Build history of the part. All positions in model axes, mm. Face numbers are marked on the shaded views. Round coordinates to 2 decimals unless told otherwise and drop trailing zeros. Order: outer loops, then holes, each group sorted by start corner. A loop starts at its lowest first (then second) coordinate and runs counter-clockwise, first axis right, second up. Notation, with made-up numbers: (-8.75, -35) -> (6.25, -35) arc R7 ccw to (6.25, -31) -> close; hole circle Ø8 at (33.25, 61). An arc over 180 degrees is marked (long way). Answer as CSV lines item,"result". Start each with the question number.
```python
from build123d import *

# Parameters (mm, degrees)
SKETCH1_R           = 5.159375
BASE_EXTRUDE_DEPTH  = 6.35
SKETCH2_R           = 20.6375
BOSS_EXTRUDE1_DEPTH = 22.225
BOSS_EXTRUDE1_TAPER = 3
SKETCH3_R           = 9.525
CUT_EXTRUDE1_DEPTH  = 52.219943931
SKETCH4_R           = 11.1125
SKETCH4_R_2         = 9.525
BOSS_EXTRUDE2_DEPTH = 0.0254
BOSS_EXTRUDE2_DRAFT = 15
SKETCH5_R           = 11.1125
CUT_EXTRUDE2_DEPTH  = 0.79375
FILLET1_R           = 1.42875


with BuildPart() as part:
    # Sketch1 → Base-Extrude (new body)
    with BuildSketch(Plane(origin=(0, 0, 0), x_dir=(0, 0, -1), z_dir=(1, 0, 0))):
        with BuildLine():
            Line((-7.223125, -19.332171929), (-35.08375, -8.92254089))
            ThreePointArc((-35.08375, -8.92254089), (-41.275, 0), (-35.08375, 8.92254089))
            Line((-35.08375, 8.92254089), (-7.223125, 19.332171929))
            ThreePointArc((-7.223125, 19.332171929), (0, 20.6375), (7.223125, 19.332171929))
            Line((7.223125, 19.332171929), (35.08375, 8.92254089))
            ThreePointArc((35.08375, 8.92254089), (41.275, 0), (35.08375, -8.92254089))
            Line((35.08375, -8.92254089), (7.223125, -19.332171929))
            ThreePointArc((7.223125, -19.332171929), (0, -20.6375), (-7.223125, -19.332171929))
        make_face()
        with Locations((-31.75, 0)):
            Circle(SKETCH1_R, mode=Mode.SUBTRACT)
        with Locations((31.75, 0)):
            Circle(SKETCH1_R, mode=Mode.SUBTRACT)
    extrude(amount=-BASE_EXTRUDE_DEPTH)

    # Sketch2 → Boss-Extrude1 (add)
    with BuildSketch(Plane.ZY):
        Circle(SKETCH2_R)
    extrude(amount=BOSS_EXTRUDE1_DEPTH, taper=BOSS_EXTRUDE1_TAPER)

    # Sketch3 → Cut-Extrude1 (cut, through all)
    with BuildSketch(Plane.ZY.offset(22.225)):
        Circle(SKETCH3_R)
    extrude(amount=-CUT_EXTRUDE1_DEPTH, mode=Mode.SUBTRACT)


with BuildPart() as boss_extrude2_tool:
    # Sketch4 → Boss-Extrude2 (with draft: the straight prism first)
    with BuildSketch(Plane.ZY.offset(22.225)):
        Circle(SKETCH4_R)
        Circle(SKETCH4_R_2, mode=Mode.SUBTRACT)
    extrude(amount=BOSS_EXTRUDE2_DEPTH)
    # Boss-Extrude2: the draft: its side faces are tilted about the plane it starts from
    boss_extrude2_sides = [boss_extrude2_tool.faces().sort_by_distance(p)[0] for p in [
        (-22.2377, 0, -11.1125),
        (-22.2377, 0, -9.525),
    ]]
    draft(boss_extrude2_sides, Plane.ZY.offset(22.225), BOSS_EXTRUDE2_DRAFT)


with BuildPart() as part_1:
    add(part.part)

    # Boss-Extrude2: add boss_extrude2_tool
    add(boss_extrude2_tool.part)

    # Sketch5 → Cut-Extrude2 (cut)
    with BuildSketch(Plane(origin=(0, 0, 0), x_dir=(0, 0, -1), z_dir=(1, 0, 0))):
        Circle(SKETCH5_R)
    extrude(amount=-CUT_EXTRUDE2_DEPTH, mode=Mode.SUBTRACT)

    # Fillet1
    fillet1_edges = [part_1.edges().sort_by_distance(p)[0] for p in [
        (-22.225, 0, -19.472737105),
    ]]
    fillet(fillet1_edges, radius=FILLET1_R)


solid = part_1.part
```
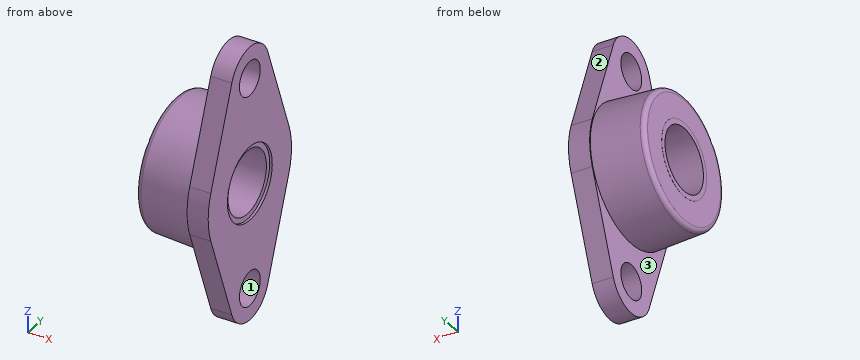
Q1. Two-plate mould, pull along Z, no slides. Class the marked faces 1, 2 and 3: +Z half, -Z half, draft (parallel to the pull), parting line (faces both ways), or undercut.
Q2. Slice it at B-B, the plane x = -5. Count the separate pieces of the cut face and the enclosed holes in it, plus the area to 3 significant figures.
Q3. Probe L1, parallel to Z at x = -4.75, y = 3.5; L2, parallel to Z at x = -5, y = 3; L3, parallel to X at y = -8, z = 29. List the from-to ranges inside material, lowest first.
Q4. Flat gauge pins, fed straight in: pin 1 Ø1.5 at (x, z) = (-19.5, -10.5) entering from +Y; pin 2 Ø2 at (x, z) = (-2.5, -19) entering from +Y; pin 3 Ø10 at (x, z) = (-16.5, 5.5) entering from +Y. Where does each tip first touch, or does it go through?
Q5. Slice it at D-D, the plane x = -13.5. Write the cut outline in (y, z) (3 decimals).
Solutions:
1,face 1,"undercut"
1,face 2,"+Z half"
1,face 3,"draft"
2,separate pieces,"1"
2,enclosed holes,"3"
2,area,"1,870 mm2"
3,L1,"z = -40.61 to -35.54, -27.96 to -8.86, 8.86 to 27.96, 35.54 to 40.61"
3,L2,"z = -40.79 to -35.95, -27.55 to -9.04, 9.04 to 27.55, 35.95 to 40.79"
3,L3,"x = -6.35 to 0"
4,pin 1,"stops at y = 17.02"
4,pin 2,"stops at y = 15.31"
4,pin 3,"stops at y = 19.87"
5,outline,"circle Ø39.86 at (0, 0); hole circle Ø19.05 at (0, 0)"
